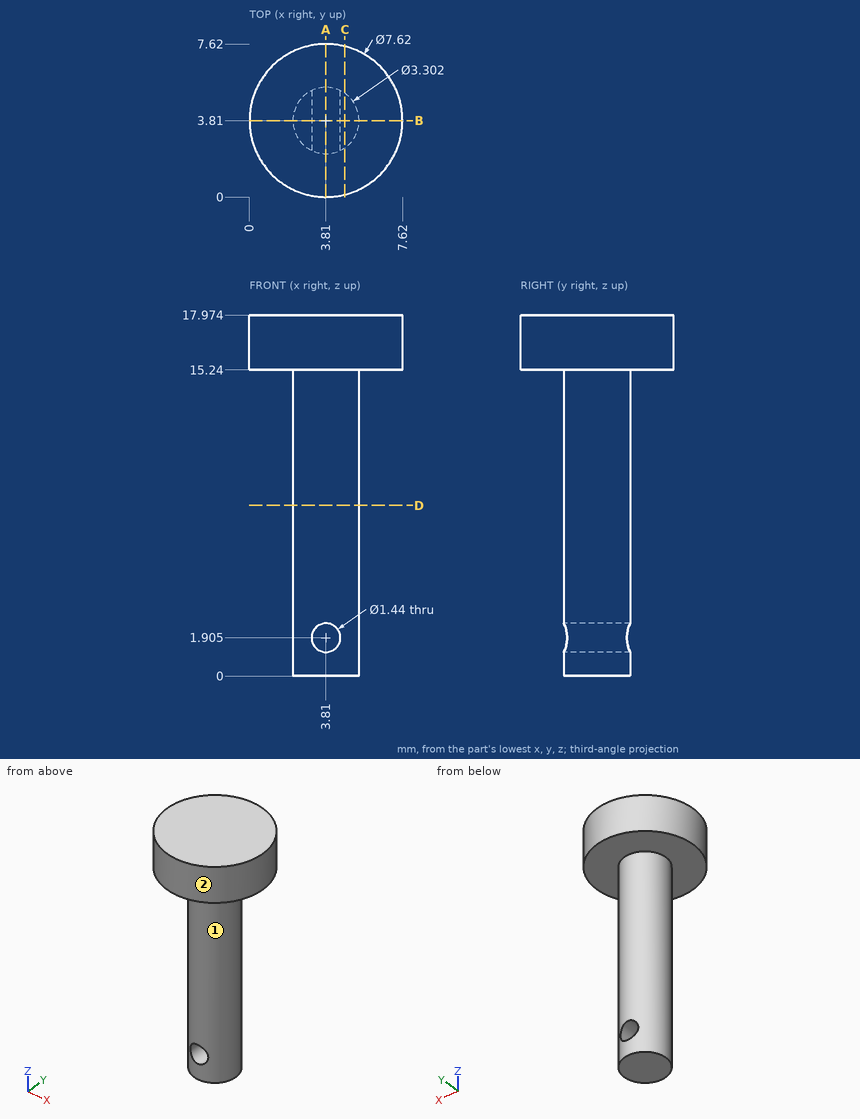
Here's the drawing with two shaded views (mm, measured from the low corner). I have some questions. A direction names the side the tool comes from. Give positions to 0.01 mm unless a question says otherwise; leave off trailing zeros. Write each loop counter-clockwise with the first axis right and the second up, starting at its lowest first coordinate (ties: lowest second). Pieces come first, ordered by that corner, then holes. Notation, with made-up numbers: (85, 86.25) -> (131, 86.25) arc R31 ccw to (131, 119.25) -> close; hole circle Ø6 at (39.5, 43.5). An arc over 180 degrees is marked (long way). Answer as a JSON object with one key per item and string values. Group by question number.
Item 1: Suppose I cut it at A-A (x = 3.81). Please give me the cut outline in (y, z) (1 decimal).
Item 2: Suppose I cut it at D-D (z = 8.5). Please give me the cut outline in (x, y).
Item 3: Suppose I cut it at B-B (y = 3.81). Please give me the cut outline in (x, z) (1 decimal).
Item 4: Please list where these lines run through material, in increasing order: line 1 (Z direction, x = 3.81, y = 4.7) (1 decimal); line 2 (Z direction, x = 1.5, y = 2); line 3 (Z direction, x = 3.25, y = 4.5) (1 decimal). Write a range as [from, to].
Item 5: I'm going to push flat-ended pins straight in: P1, Ø1.7, axis at x = 3.81, z = 1.905, coming from the -Y side; P2, Ø2, axis at x = 2, z = 13, coming from the +Y side; P3, Ø1, axis at y = 4, z = 6, coming from the -X side. Where does each tip first touch, or does it pass through?
Item 6: For the marked faces 1 and 2, which set-ups out of +Z, -Z, +X, -X, +Y, -Y let a thin tool reach every point of the face, with its end or its side?
Item 7: Suppose I cut it at C-C (x = 4.75). Please give me the cut outline in (y, z).
Findings:
{
 "1": {"outline": "(0, 15.2) -> (2.2, 15.2) -> (2.2, 2.6) -> (5.5, 2.6) -> (5.5, 15.2) -> (7.6, 15.2) -> (7.6, 18) -> (0, 18) -> close; (2.2, 0) -> (5.5, 0) -> (5.5, 1.2) -> (2.2, 1.2) -> close"},
 "2": {"outline": "circle Ø3.3 at (3.81, 3.81)"},
 "3": {"outline": "(0, 15.2) -> (2.2, 15.2) -> (2.2, 0) -> (5.5, 0) -> (5.5, 15.2) -> (7.6, 15.2) -> (7.6, 18) -> (0, 18) -> close; hole circle Ø1.4 at (3.8, 1.9)"},
 "4": {"line 1": "z = [0, 1.2], [2.6, 18]", "line 2": "z = [15.24, 17.97]", "line 3": "z = [0, 1.5], [2.4, 18]"},
 "5": {"P1": "stops at y = 2.16", "P2": "stops at y = 5.25", "P3": "stops at x = 2.16"},
 "6": {"face 1": "-Z", "face 2": "+Z, -Z"},
 "7": {"outline": "(0.12, 15.24) -> (2.45, 15.24) -> (2.45, 0) -> (5.17, 0) -> (5.17, 15.24) -> (7.5, 15.24) -> (7.5, 17.97) -> (0.12, 17.97) -> close"}
}
